Part model, mm, in its own coordinate system. A direction names the side the tool comes from. Round coordinates to 2 decimals unless told otherwise and drop trailing zeros. Write each loop counter-clockwise with the first axis right and the second up, starting at its lowest first coordinate (ties: lowest second). Pieces come first, ordered by that corner, then holes. Notation, with made-up numbers: M 9.25,17.5 L 58.25,17.5 A35 ccw 58.25,52.5 Z; hole C -38,42.5 d2. An arc over 180 degrees is marked long. Use a Markdown table: item, result. Add a question column.
1) Slice it at A-A on z = 2. Write the cut outline in (x, y), plus the area to 3 significant figures.
2) Drop flat-ended pins along their axis: P1, Ø2.5, axis at y = -12, z = 25, coming from the -X side; P2, Ø3, axis at x = 20, y = -13.5, coming from the -Z side; P3, Ø1.1, axis at x = 14, y = -3, coming from the +Z side. Give the stop position or say it passes through.
3) Slice it at D-D on x = -8. Write the cut outline in (y, z).
4) Which spindle directions (+Z, -Z, +X, -X, +Y, -Y) get a long thin tool onto all of the face, cutting with end or side? Do faces 1 (the face through (19, -12, -21)), 2 (the face through (6.5, -1, 28)), 3 (the face through (7.33, -0.14, 21.65)). Say none if no direction does.
5) Slice it at B-B on y = -12. Write the cut outline in (x, z), plus the area to 3 significant figures.
6) Slice it at C-C on x = 10.5. Write the cut outline in (y, z), plus the area to 3 significant figures.
7) Two-plate mould, pull along X, no slides. Class faces 4 (the face through (10.703, -12.288, -22.141)), 5 (the face through (-11.5, -7, 0)), 6 (the face through (13.03, -0.36, 9.3)): released by +X, released by -X, zero draft, split by the parting line, or undercut.
8) Wall check: probe 1 along Z at (x, y) = (-9.05, -12); probe 2 along Y at (x, z) = (-7.15, -25); probe 3 along X at (y, z) = (-14.25, -13). Give the ranges that are in metal, low to high.
```python
from build123d import *

# Parameters (mm, degrees)
F0_W           = 21
F0_H           = 66
F0_W_2         = 11
F0_H_2         = 56.642
F1_DEPTH       = 15
F2_R           = 5
F4_START       = 9.5
F3_W           = 15
F3_H           = 42
F4_DEPTH       = 5.5
F5_T1_DEPTH    = 15
F6_W           = 1.5
F6_H           = 6.5
F7_DEPTH       = 50
F7_DEPTH_BACK  = 50
F8_R           = 1.5
F9_DEPTH       = 5
F10_W          = 3
F10_H          = 1
F11_DEPTH      = 33
F11_DEPTH_BACK = 33
F12_SIZE       = 0.5
F13_W          = 5
F13_H          = 12
F14_DEPTH      = 14
F15_R          = 4
F16_W          = 13
F16_H          = 70
F17_DEPTH      = 2
F18_W          = 20
F18_H          = 12
F19_DEPTH      = 2
F20_R          = 2
F21_T1_DEPTH   = 68.8536746712
F21_T3_DEPTH   = 11.490341494
F21_T5_DEPTH   = 3
F21_T7_DEPTH   = 8
F21_T9_DEPTH   = 11.490341494
F21_T11_DEPTH  = 13.591
F21_T13_DEPTH  = 8
F21_T16_ANGLE  = 90
F21_T18_ANGLE  = 90
F21_T20_ANGLE  = 90
F21_T22_ANGLE  = 90
F21_T24_ANGLE  = 90
F21_T26_ANGLE  = 90
F21_T28_ANGLE  = 90
F21_T30_ANGLE  = 90
F23_START      = -6.5
F22_R          = 6
F23_DEPTH      = 5.001


# Not quite as in the source:
# - a fillet or chamfer that OpenCascade refuses, or shapes differently, is made with other operations: its cross-section is extruded or revolved along the edge and cut away or added


with BuildPart() as f1:
    # F0 (on Front) → F1 (new body)
    with BuildSketch(Plane.XZ):
        with Locations((-1, 0)):
            Rectangle(F0_W, F0_H)
        Rectangle(F0_W_2, F0_H_2, mode=Mode.SUBTRACT)
    extrude(amount=F1_DEPTH)

    # F2
    f2_edges = [f1.edges().sort_by_distance(p)[0] for p in [
        (-11.5, 0, 0),
    ]]
    fillet(f2_edges, radius=F2_R)

    # F3 (on Front) → F4 (join)
    with BuildSketch(Plane.XZ.offset(F4_START)):
        with Locations((17, 0)):
            Rectangle(F3_W, F3_H)
    extrude(amount=F4_DEPTH)

    # F5: fillet of radius 2 on 4 edges, made by hand

    # F5_s2 → F5_t1 (join)
    with BuildSketch(Plane.XZ):
        with BuildLine():
            ThreePointArc((5.5001, -26.3211), (4.9143135624, -27.7353135624), (3.5001, -28.3211))
            Line((3.5001, -28.3211), (3.5001, -28.3611))
            ThreePointArc((3.5001, -28.3611), (4.50005, -28.361), (5.5, -28.361))
            Line((5.5, -28.361), (5.54, -28.321))
            ThreePointArc((5.54, -28.321), (5.54, -27.32105), (5.5401, -26.3211))
            Line((5.5401, -26.3211), (5.5001, -26.3211))
        make_face()
        with BuildLine():
            ThreePointArc((-3.5001, -28.3211), (-4.9143135624, -27.7353135624), (-5.5001, -26.3211))
            Line((-5.5001, -26.3211), (-5.5401, -26.3211))
            ThreePointArc((-5.5401, -26.3211), (-5.54, -27.32105), (-5.54, -28.321))
            Line((-5.54, -28.321), (-5.5, -28.361))
            ThreePointArc((-5.5, -28.361), (-4.50005, -28.361), (-3.5001, -28.3611))
            Line((-3.5001, -28.3611), (-3.5001, -28.3211))
        make_face()
        with BuildLine():
            ThreePointArc((-5.5001, 26.3211), (-4.9143135624, 27.7353135624), (-3.5001, 28.3211))
            Line((-3.5001, 28.3211), (-3.5001, 28.3611))
            ThreePointArc((-3.5001, 28.3611), (-4.50005, 28.361), (-5.5, 28.361))
            Line((-5.5, 28.361), (-5.54, 28.321))
            ThreePointArc((-5.54, 28.321), (-5.54, 27.32105), (-5.5401, 26.3211))
            Line((-5.5401, 26.3211), (-5.5001, 26.3211))
        make_face()
        with BuildLine():
            ThreePointArc((5.5001, 26.3211), (4.9143135624, 27.7353135624), (3.5001, 28.3211))
            Line((3.5001, 28.3211), (3.5001, 28.3611))
            ThreePointArc((3.5001, 28.3611), (4.50005, 28.361), (5.5, 28.361))
            Line((5.5, 28.361), (5.54, 28.321))
            ThreePointArc((5.54, 28.321), (5.54, 27.32105), (5.5401, 26.3211))
            Line((5.5401, 26.3211), (5.5001, 26.3211))
        make_face()
    extrude(amount=F5_T1_DEPTH)

    # F6 (on Top) → F7 (cut, two sides)
    with BuildSketch(Plane.XY) as f7_sk:
        with Locations((-10.75, -11.75)):
            Rectangle(F6_W, F6_H)
    extrude(amount=-F7_DEPTH, mode=Mode.SUBTRACT)
    extrude(f7_sk.sketch, amount=F7_DEPTH_BACK, mode=Mode.SUBTRACT)

    # F8 (on face) → F9 (cut)
    with BuildSketch(Plane(origin=(-10, 0, 0), x_dir=(0, -1, 0), z_dir=(-1, 0, 0))):
        with Locations((12, 25)):
            Circle(F8_R)
        with Locations((12, -25)):
            Circle(F8_R)
    extrude(amount=-F9_DEPTH, mode=Mode.SUBTRACT)

    # F10 (on Top) → F11 (join, two sides)
    with BuildSketch(Plane.XY) as f11_sk:
        with Locations((16, -0.5)):
            Rectangle(F10_W, F10_H)
        Polygon((14.5, -5.45), (14.5, -1), (14.5, 0), (9.5, 0), (9.5, -5.45), align=None)
    extrude(amount=F11_DEPTH)
    extrude(f11_sk.sketch, amount=-F11_DEPTH_BACK)

    # F12
    f12_edges = [f1.edges().sort_by_distance(p)[0] for p in [
        (17.5, 0, 0),
    ]]
    chamfer(f12_edges, length=F12_SIZE)

    # F13 (on face) → F14 (cut)
    with BuildSketch(Plane.XZ.offset(15)):
        with Locations((12, -27)):
            Rectangle(F13_W, F13_H)
        with Locations((12, 27)):
            Rectangle(F13_W, F13_H)
    extrude(amount=-F14_DEPTH, mode=Mode.SUBTRACT)

    # F15
    f15_edges = [f1.edges().sort_by_distance(p)[0] for p in [
        (9.5, -3.225, -21),
        (9.5, -12.25, -21),
        (9.5, -3.225, 21),
        (9.5, -12.25, 21),
    ]]
    fillet(f15_edges, radius=F15_R)

    # F16 (on Front) → F17 (cut)
    with BuildSketch(Plane.XZ):
        Rectangle(F16_W, F16_H)
    extrude(amount=F17_DEPTH, mode=Mode.SUBTRACT)

    # F18 (on face) → F19 (cut)
    with BuildSketch(Plane(origin=(0, 0, 0), x_dir=(-1, 0, 0), z_dir=(0, 1, 0))):
        with Locations((-3.5, 14.7955)):
            Rectangle(F18_W, F18_H)
        with Locations((-3.5, -14.7955)):
            Rectangle(F18_W, F18_H)
    extrude(amount=-F19_DEPTH, mode=Mode.SUBTRACT)

    # F20
    f20_edges = [f1.edges().sort_by_distance(p)[0] for p in [
        (13.5, -1, -20.7955),
        (13.5, -1, 20.7955),
        (6.5, -1, 20.7955),
        (6.5, -1, 8.7955),
        (6.5, -1, -8.7955),
        (6.5, -1, -20.7955),
        (13.5, -1, -8.7955),
        (13.5, -1, 8.7955),
    ]]
    fillet(f20_edges, radius=F20_R)

    # F21: chamfer of 0.5 on 18 edges, made by hand

    # F21_s2 → F21_t1 (cut)
    with BuildSketch(Plane.XY.offset(-34.4268373356)):
        with BuildLine():
            Line((-7.0555555556, -0.03096005), (-6.5, -0.527864045))
            Line((-6.5, -0.527864045), (-6.5, 0))
            ThreePointArc((-6.5, 0), (-6.7852695606, -0.0081445055), (-7.0555555556, -0.03096005))
        make_face()
    extrude(amount=F21_T1_DEPTH, mode=Mode.SUBTRACT)

    # F21_s4 → F21_t3 (cut)
    with BuildSketch(Plane.XY.offset(-34.285841494)):
        Polygon((7, 0), (6.5, -0.5), (6.5, 0), align=None)
    extrude(amount=F21_T3_DEPTH, mode=Mode.SUBTRACT)

    # F21_s6 → F21_t5 (cut)
    with BuildSketch(Plane.YZ.offset(8.5)):
        Polygon((0, -21.2955), (-0.5, -20.7955), (0, -20.7955), align=None)
        Polygon((0, -8.2955), (-0.5, -8.7955), (0, -8.7955), align=None)
        Polygon((0, 21.2955), (-0.5, 20.7955), (0, 20.7955), align=None)
        Polygon((0, 8.2955), (-0.5, 8.7955), (0, 8.7955), align=None)
    extrude(amount=F21_T5_DEPTH, mode=Mode.SUBTRACT)

    # F21_s8 → F21_t7 (cut)
    with BuildSketch(Plane.XY.offset(-18.7955)):
        Polygon((14, 0), (13.5, -0.5), (13.5, 0), align=None)
    extrude(amount=F21_T7_DEPTH, mode=Mode.SUBTRACT)

    # F21_s10 → F21_t9 (cut)
    with BuildSketch(Plane.XY.offset(22.7955)):
        Polygon((7, 0), (6.5, -0.5), (6.5, 0), align=None)
    extrude(amount=F21_T9_DEPTH, mode=Mode.SUBTRACT)

    # F21_s12 → F21_t11 (cut)
    with BuildSketch(Plane.XY.offset(-6.7955)):
        Polygon((7, 0), (6.5, -0.5), (6.5, 0), align=None)
    extrude(amount=F21_T11_DEPTH, mode=Mode.SUBTRACT)

    # F21_s14 → F21_t13 (cut)
    with BuildSketch(Plane.XY.offset(10.7955)):
        Polygon((14, 0), (13.5, -0.5), (13.5, 0), align=None)
    extrude(amount=F21_T13_DEPTH, mode=Mode.SUBTRACT)

    # F21_s15 → F21_t16 (revolve, cut)
    with BuildSketch(Plane.YZ.offset(8.5)):
        Polygon((0, -21.2955), (-0.5, -20.7955), (0, -20.7955), align=None)
    revolve(axis=Axis((8.5, 0, -22.7955), (0, -1, 0)), revolution_arc=F21_T16_ANGLE, mode=Mode.SUBTRACT)

    # F21_s17 → F21_t18 (revolve, cut)
    with BuildSketch(Plane.XY.offset(-18.7955)):
        Polygon((14, 0), (13.5, -0.5), (13.5, 0), align=None)
    revolve(axis=Axis((11.5, 0, -18.7955), (0, 1, 0)), revolution_arc=F21_T18_ANGLE, mode=Mode.SUBTRACT)

    # F21_s19 → F21_t20 (revolve, cut)
    with BuildSketch(Plane.YZ.offset(11.5)):
        Polygon((0, -8.2955), (-0.5, -8.7955), (0, -8.7955), align=None)
    revolve(axis=Axis((11.5, 0, -10.7955), (0, 1, 0)), revolution_arc=F21_T20_ANGLE, mode=Mode.SUBTRACT)

    # F21_s21 → F21_t22 (revolve, cut)
    with BuildSketch(Plane.XY.offset(22.7955)):
        Polygon((7, 0), (6.5, -0.5), (6.5, 0), align=None)
    revolve(axis=Axis((8.5, 0, 22.7955), (0, -1, 0)), revolution_arc=F21_T22_ANGLE, mode=Mode.SUBTRACT)

    # F21_s23 → F21_t24 (revolve, cut)
    with BuildSketch(Plane.XY.offset(-6.7955)):
        Polygon((7, 0), (6.5, -0.5), (6.5, 0), align=None)
    revolve(axis=Axis((8.5, 0, -6.7955), (0, -1, 0)), revolution_arc=F21_T24_ANGLE, mode=Mode.SUBTRACT)

    # F21_s25 → F21_t26 (revolve, cut)
    with BuildSketch(Plane.YZ.offset(11.5)):
        Polygon((0, 21.2955), (-0.5, 20.7955), (0, 20.7955), align=None)
    revolve(axis=Axis((11.5, 0, 18.7955), (0, 1, 0)), revolution_arc=F21_T26_ANGLE, mode=Mode.SUBTRACT)

    # F21_s27 → F21_t28 (revolve, cut)
    with BuildSketch(Plane.YZ.offset(8.5)):
        Polygon((0, 8.2955), (-0.5, 8.7955), (0, 8.7955), align=None)
    revolve(axis=Axis((8.5, 0, 6.7955), (0, -1, 0)), revolution_arc=F21_T28_ANGLE, mode=Mode.SUBTRACT)

    # F21_s29 → F21_t30 (revolve, cut)
    with BuildSketch(Plane.XY.offset(10.7955)):
        Polygon((14, 0), (13.5, -0.5), (13.5, 0), align=None)
    revolve(axis=Axis((11.5, 0, 10.7955), (0, 1, 0)), revolution_arc=F21_T30_ANGLE, mode=Mode.SUBTRACT)

    # F22 (on Right) → F23 (cut)
    with BuildSketch(Plane.YZ.offset(F23_START)):
        with Locations((3, -14.7955)):
            Circle(F22_R)
        with Locations((3, 14.7955)):
            Circle(F22_R)
    extrude(amount=-F23_DEPTH, mode=Mode.SUBTRACT)


solid = f1.part
```
Entries:
| question | item | result |
|---|---|---|
| 1 | outline | M -11.5,-8.5 L -10,-8.5 L -10,-15 L -5.5,-15 L -5.5,-2 L -6.5,-2 L -6.5,-0.53 L -7.06,-0.03 A5 ccw -11.5,-5 Z; M 5.5,-15 L 24.5,-15 L 24.5,-9.5 L 9.5,-9.5 L 9.5,-5.45 L 14.5,-5.45 L 14.5,-1 L 17.5,-1 L 17.5,-0.5 L 17,0 L 7,0 L 6.5,-0.5 L 6.5,-2 L 5.5,-2 Z |
| 1 | area | 243 mm^2 |
| 2 | P1 | stops at x = 5.5 |
| 2 | P2 | stops at z = -21 |
| 2 | P3 | stops at z = 21 |
| 3 | outline | M -15,-33 L -0.23,-33 L -0.23,-19.85 A6 cw -0.23,-9.74 L -0.23,9.74 A6 cw -0.23,19.85 L -0.23,33 L -15,33 Z; hole C -12,-25 d3; hole C -12,25 d3 |
| 4 | face 1 | -Z, +X, -Y |
| 4 | face 2 | +Z, -Z, +Y |
| 4 | face 3 | +Y |
| 5 | outline | M -10,-33 L 9.5,-33 L 9.5,-25 A4 cw 13.5,-21 L 24.5,-21 L 24.5,21 L 13.5,21 A4 cw 9.5,25 L 9.5,33 L -10,33 L -10,26.5 L -5.49,26.5 A2 cw -3.52,28.32 L 3.52,28.32 A2 cw 5.5,26.34 L 5.5,-26.34 A2 cw 3.52,-28.32 L -3.52,-28.32 A2 cw -5.49,-26.5 L -10,-26.5 Z; M -10,-23.5 L -5.5,-23.5 L -5.5,23.5 L -10,23.5 Z |
| 5 | area | 1,280 mm^2 |
| 6 | outline | M -15,-22.35 L -9.5,-22.35 L -9.5,22.35 L -15,22.35 Z; M -5.45,-22.35 L -1,-22.35 L -1,-33 L 0,-33 L 0,-21.3 L -0.5,-20.8 L -2,-20.8 L -2,-8.8 L -0.5,-8.8 L 0,-8.3 L 0,8.3 L -0.5,8.8 L -2,8.8 L -2,20.8 L -0.5,20.8 L 0,21.3 L 0,33 L -1,33 L -1,22.35 L -5.45,22.35 Z |
| 6 | area | 462 mm^2 |
| 7 | face 4 | released by +X |
| 7 | face 5 | released by -X |
| 7 | face 6 | undercut |
| 8 | probe 1 | z = -33 to -26.5, -23.5 to 23.5, 26.5 to 33 |
| 8 | probe 2 | y = -15 to -13.5, -10.5 to -0.04 |
| 8 | probe 3 | x = -10 to -5.5, 5.5 to 24.5 |
